from build123d import *

# Parameters (mm, degrees)
SKETCH1_W           = 32.3
SKETCH1_H           = 18.6
BOSS_EXTRUDE1_DEPTH = 1.8
SKETCH5_W           = 7
SKETCH5_H           = 18.6
BOSS_EXTRUDE3_DEPTH = 0.8
SKETCH6_R           = 1.75
CUT_EXTRUDE3_DEPTH  = 0.8


with BuildPart() as part:
    # Sketch1 → Boss-Extrude1 (new body)
    with BuildSketch(Plane.XY):
        Rectangle(SKETCH1_W, SKETCH1_H)
    extrude(amount=BOSS_EXTRUDE1_DEPTH)

    # Sketch5 → Boss-Extrude3 (add)
    with BuildSketch(Plane.XY.offset(1.8)):
        with Locations((-19.65, 0)):
            Rectangle(SKETCH5_W, SKETCH5_H)
        with Locations((19.65, 0)):
            Rectangle(SKETCH5_W, SKETCH5_H)
    extrude(amount=-BOSS_EXTRUDE3_DEPTH)

    # Sketch6 → Cut-Extrude3 (cut)
    with BuildSketch(Plane.XY.offset(1.8)):
        with Locations((-19.65, 0)):
            Circle(SKETCH6_R)
        with Locations((19.65, 0)):
            Circle(SKETCH6_R)
    extrude(amount=-CUT_EXTRUDE3_DEPTH, mode=Mode.SUBTRACT)


solid = part.part
Check sheet for the modelled part. Datum: model origin and axes. Units: mm. A direction names the side the tool comes from. Round coordinates to 2 decimals unless told otherwise and drop trailing zeros. Loops run counter-clockwise (first coordinate to the right, second up) from the corner with the lowest first, then second, coordinate; pieces in that order, holes last. Notation, with made-up numbers: (22.5, 17) - (80.5, 17) arc R28 cw to (80.5, 44) - close; hole circle Ø8 at (-18, -26.5). An arc over 180 degrees is marked (long way). Answer as CSV lines item,"result". Start each with the question number.
Item 1: Section check D-D (y = 2.75). Record the boundary of the cut face in (x, z).
Item 2: Section check C-C (z = 1.5). Record the boundary of the cut face in (x, y), and give its area (3 significant figures).
Item 3: Section check B-B (y = 0). Record the boundary of the cut face in (x, z).
Item 4: Section check A-A (x = -19.65). Record the boundary of the cut face in (y, z), and give its area (3 significant figures).
Item 5: Scan lines: line 1 (Y direction, x = 19.65, z = 1.5); line 2 (X direction, y = 0.25, z = 1.25); line 3 (X direction, y = -1.5, z = 0.8). Record each from-to range of solid material in increasing order. Write a range as [from, to].
Item 6: Set-up check for faces 1 (the flat face through (16.15, -0.1, 0.5)), 2 (the flat face through (0, 9.3, 1)), 3 (the flat face through (-20, 2, 1)): record each of +Z, -Z, +X, -X, +Y, -Y from which the full face is reachable in a straight line by a thin tool's end or side.
Item 7: Depth check by flat-ended pin: P1, Ø5.5, axis at x = -19.65, y = 0, coming from the -Z side; P2, Ø0.5, axis at y = -1.5, z = 0.5, coming from the +X side; P3, Ø3, axis at x = 19.65, y = 0, coming from the -Z side. Enter the tip coordinate at first touch or a pass-through.
Item 8: Release check for a two-part mould opening along Y. For faces 4 (the cylindrical face through (-17.981, 0.526, 1.406)), 5 (the flat face through (0, -9.3, 1)), 6 (the flat face through (-16.15, -0.1, 0.5)) record: +Y half, -Y half, draft (parallel to the pull), parting line (faces both ways), or undercut.
Report:
1,outline,"(-23.15, 1) - (-16.15, 1) - (-16.15, 0) - (16.15, 0) - (16.15, 1) - (23.15, 1) - (23.15, 1.8) - (-23.15, 1.8) - close"
2,outline,"(-23.15, -9.3) - (23.15, -9.3) - (23.15, 9.3) - (-23.15, 9.3) - close; hole circle Ø3.5 at (-19.65, 0); hole circle Ø3.5 at (19.65, 0)"
2,area,"842 mm2"
3,outline,"(-23.15, 1) - (-21.4, 1) - (-21.4, 1.8) - (-23.15, 1.8) - close; (-17.9, 1) - (-16.15, 1) - (-16.15, 0) - (16.15, 0) - (16.15, 1) - (17.9, 1) - (17.9, 1.8) - (-17.9, 1.8) - close; (21.4, 1) - (23.15, 1) - (23.15, 1.8) - (21.4, 1.8) - close"
4,outline,"(-9.3, 1) - (-1.75, 1) - (-1.75, 1.8) - (-9.3, 1.8) - close; (1.75, 1) - (9.3, 1) - (9.3, 1.8) - (1.75, 1.8) - close"
4,area,"12.1 mm2"
5,line 1,"y = [-9.3, -1.75], [1.75, 9.3]"
5,line 2,"x = [-23.15, -21.38], [-17.92, 17.92], [21.38, 23.15]"
5,line 3,"x = [-16.15, 16.15]"
6,face 1,"-Z, +X, +Y, -Y"
6,face 2,"+Z, -Z, +X, -X, +Y"
6,face 3,"-Z, -X, +Y, -Y"
7,P1,"stops at z = 1"
7,P2,"stops at x = 16.15"
7,P3,"passes through"
8,face 4,"undercut"
8,face 5,"-Y half"
8,face 6,"draft"
